Autodesk Fusion 360 part; units mm, degrees
sketch "Esquisse1" plane through (0, 0, 0) normal (0, 1, 0) x (1, 0, 0)
  circle A0 centre (0, 0) radius 12
  line L0 (0, 0) -> (0, 12)
  circle A1 centre (0, 0) radius 9
  circle A2 centre (0, 9) radius 1.6
  circle A3 centre (-7.7942, -4.5) radius 1.6
  circle A4 centre (7.7942, -4.5) radius 1.6
  dimension "d1" = 24
  dimension "d2" = 18
  dimension "d3" = 3.2
  dimension "d5" = 360
extrude "Extrusion1" add sketch "Esquisse1" along normal blind 1.2 contours A0 | A1 A2 A3 A4 makes body 1
sketch "Esquisse2" plane through (0, 1.2, 0) normal (0, 1, 0) x (-1, 0, 0)
  circle A0 centre (-7.7942, 4.5) radius 1.6
  circle A1 centre (0, -9) radius 1.6
  circle A2 centre (7.7942, 4.5) radius 1.6
  circle A3 centre (0, 0) radius 12
  circle A4 centre (0, 0) radius 6.25
  dimension "d8" = 12.5
extrude "Extrusion2" add sketch "Esquisse2" along normal blind 5 contours A4 bodies 1
sketch "Esquisse3" plane through (0, 0, 0) normal (0, -1, 0) x (1, 0, 0)
  circle A0 centre (7.7942, 4.5) radius 1.6
  circle A1 centre (0, -9) radius 1.6
  circle A2 centre (-7.7942, 4.5) radius 1.6
  circle A3 centre (0, 0) radius 12
  circle A4 centre (0, 0) radius 6.25
  dimension "d11" = 12.5
extrude "Extrusion3" add sketch "Esquisse3" along normal blind 15.4 contours A4 bodies 1
sketch "Esquisse4" plane through (0, 6.2, 0) normal (0, 1, 0) x (-1, 0, 0)
  circle A0 centre (0, 0) radius 6.25
  circle A1 centre (0, 0) radius 2.5
  dimension "d14" = 5
extrude "Extrusion4" add sketch "Esquisse4" along normal blind 1.5 contours A1 bodies 1
copy_body "Corps->Comp1" bodies 1 removing the originals makes body 2 in component "anneau coulissant rotatif"
component "anneau coulissant rotatif" placed x (1, 0, 0) y (0, 1, 0) z (0, 0, 1) at (0, 0, 0)
equation "d12 = 21.6 mm - 5 mm - 1.2 mm"
Part model, mm, in its own coordinate system. A direction names the side the tool comes from. Give positions to 0.01 mm unless a question says otherwise; leave off trailing zeros. Loops run counter-clockwise (first coordinate to the right, second up) from the corner with the lowest first, then second, coordinate; pieces in that order, holes last. Notation, with made-up numbers: M 44.5,37 L 54.5,37 A17 ccw 54.5,65 Z; hole C 30.5,-20 d6. An arc over 180 degrees is marked long. Put each result on its own line as item: value. Start each with the question number.
1) Saw through at A-A (x = 0). List the corners of the cut face in (y, z), then the cut area to 3 significant figures.
2) Probe probe 1 along Z at (x, y) = (0, 0.55); probe 2 along X at (y, z) = (0.35, 4.5); probe 3 along Y at (x, z) = (5.5, -10.5). List the from-to ranges inside material, lowest first.
3) Saw through at D-D (z = 0). List the corners of the cut face in (x, y), then the cut area to 3 significant figures.
4) Saw through at C-C (z = 4.5). List the corners of the cut face in (x, y).
5) Saw through at B-B (z = -9). List the corners of the cut face in (x, y).
6) 3-axis set-ups, long thin cutter, end or side, ignore diameter. For faces 1 (the cylindrical face through (5.96, -7.59, -1.88)), 2 (the flat face through (5, 1.2, 5)), 3 (the cylindrical face through (8.53, 0.59, 3.08)): which of +Z, -Z, +X, -X, +Y, -Y reach the whole face in a straight line?
7) Flat gauge pins, fed straight in: pin 1 (1 mm diameter, centred on x = 2, y = -12.5, fed in from -Z); pin 2 (3 mm diameter, centred on x = -9, z = 9, fed in from +Y); pin 3 (6 mm diameter, centred on x = -2, y = -4, fed in from +Z). Where does each tip first touch, or does it go through?
8) Pull direction X, two halves, no side cores. Call faces 4 (the cylindrical face through (-5.96, 3.66, -1.88)), 5 (the cylindrical face through (-6.316, 0.592, 3.887)), 6 (the cylindrical face through (-0.35, 0.59, -10.56)), 7 (the flat face through (0, -15.4, 0)): +X half, -X half, draft (parallel to the pull), parting line (faces both ways), or undercut.
Numbers:
1. outline: M -15.4,-6.25 L 0,-6.25 L 0,-7.4 L 1.2,-7.4 L 1.2,-6.25 L 6.2,-6.25 L 6.2,-2.5 L 7.7,-2.5 L 7.7,2.5 L 6.2,2.5 L 6.2,6.25 L 1.2,6.25 L 1.2,12 L 0,12 L 0,6.25 L -15.4,6.25 Z; M 0,-12 L 1.2,-12 L 1.2,-10.6 L 0,-10.6 Z
1. area: 287 mm^2
2. probe 1: -12 to -10.6, -7.4 to 12
2. probe 2: -11.12 to -9.39, -6.19 to 6.19, 9.39 to 11.12
2. probe 3: 0 to 1.2
3. outline: M -12,0 L -6.25,0 L -6.25,-15.4 L 6.25,-15.4 L 6.25,0 L 12,0 L 12,1.2 L 6.25,1.2 L 6.25,6.2 L 2.5,6.2 L 2.5,7.7 L -2.5,7.7 L -2.5,6.2 L -6.25,6.2 L -6.25,1.2 L -12,1.2 Z
3. area: 291 mm^2
4. outline: M -11.12,0 L -9.39,0 L -9.39,1.2 L -11.12,1.2 Z; M -6.19,0 L -4.34,0 L -4.34,-15.4 L 4.34,-15.4 L 4.34,0 L 6.19,0 L 6.19,1.2 L 4.34,1.2 L 4.34,6.2 L -4.34,6.2 L -4.34,1.2 L -6.19,1.2 Z; M 9.39,0 L 11.12,0 L 11.12,1.2 L 9.39,1.2 Z
5. outline: M -7.94,0 L -1.6,0 L -1.6,1.2 L -7.94,1.2 Z; M 1.6,0 L 7.94,0 L 7.94,1.2 L 1.6,1.2 Z
6. face 1: -Y
6. face 2: +Y
6. face 3: +Y, -Y
7. pin 1: z = -6.07
7. pin 2: y = 1.2
7. pin 3: z = 6.25
8. face 4: parting line
8. face 5: undercut
8. face 6: undercut
8. face 7: draft
